The model under review builds one solid part; all positions refer to its coordinate system, in mm. A direction names the side the tool comes from. Coordinates: 2 decimals unless noted, no trailing zeros. Order: outer loops, then holes, each group sorted by start corner. A loop starts at its lowest first (then second) coordinate and runs counter-clockwise, first axis right, second up. Notation, with made-up numbers: (34.25, 35.25) - (88.25, 35.25) arc R16 cw to (88.25, 42.25) - close; hole circle Ø2 at (78.5, 9). An arc over 180 degrees is marked (long way). Answer in a Markdown table with one row per item.
```python
from build123d import *

# Parameters (mm, degrees)
F0_R     = 8.75
F0_R_2   = 4
F1_DEPTH = 21.3
F2_START = 3.8
F0_R_3   = 2.65
F2_DEPTH = 17.5
F4_DEPTH = 10


with BuildPart() as f1:
    # F0 (on Top) → F1 (new body)
    with BuildSketch(Plane.XY):
        Circle(F0_R)
        Circle(F0_R_2, mode=Mode.SUBTRACT)
    extrude(amount=F1_DEPTH)

    # F0 (on Top) → F2 (join)
    with BuildSketch(Plane.XY.offset(F2_START)):
        Circle(F0_R_2)
        Circle(F0_R_3, mode=Mode.SUBTRACT)
    extrude(amount=F2_DEPTH)

    # F3 (on face) → F4 (cut)
    with BuildSketch(Plane.XY.offset(21.3)):
        with BuildLine():
            ThreePointArc((-6.8053287944, -5.5), (0, -8.75), (6.8053287944, -5.5))
            Line((6.8053287944, -5.5), (-6.8053287944, -5.5))
        make_face()
        with BuildLine():
            Line((-6.8053287944, 5.5), (6.8053287944, 5.5))
            ThreePointArc((6.8053287944, 5.5), (0, 8.75), (-6.8053287944, 5.5))
        make_face()
    extrude(amount=-F4_DEPTH, mode=Mode.SUBTRACT)


solid = f1.part
```
Item 1: Mouldability with a two-part tool opening along Y and no side actions: class faces 4 (the face through (2.45, -1.01, 12.43)), 5 (the face through (4, -2, 0)), 6 (the face through (0, 5.5, 16)) as +Y half, -Y half, draft (parallel to the pull), parting line (faces both ways), or undercut.
Check values:
| item | result |
|---|---|
| face 4 | undercut |
| face 5 | draft |
| face 6 | +Y half |
Item 2: To check wall thickness, follow line 1 (Y direction, x = 0, z = 10.5); line 2 (Y direction, x = 0, z = 2.85); line 3 (X direction, y = 5.5, z = 7). State the ranges of each line that lie inside material, in increasing order. Write a range as from..to.
Check values:
| item | result |
|---|---|
| line 1 | -8.75..-2.65, 2.65..8.75 |
| line 2 | -8.75..-4, 4..8.75 |
| line 3 | -6.81..6.81 |
Item 3: Clearance check with flat-ended pins moving along their axes: pin 1 Ø1 at (x, z) = (2, 13.5) entering from -Y; pin 2 Ø4 at (x, y) = (1.5, 1) entering from -Z; pin 3 Ø1 at (x, z) = (1, 7) entering from -Y. State where each tip first meets the part, or that it passes through.
Check values:
| item | result |
|---|---|
| pin 1 | y = -5.5 |
| pin 2 | z = 3.8 |
| pin 3 | y = -8.74 |
Item 4: We need section C-C, the plane z = 13. Write out the cut boundary in (x, y), then the cut area to 3 significant figures.
Check values:
| item | result |
|---|---|
| outline | (-6.81, -5.5) - (6.81, -5.5) arc R8.75 ccw to (6.81, 5.5) - (-6.81, 5.5) arc R8.75 ccw to start; hole circle Ø5.3 at (0, 0) |
| area | 157 mm^2 |
Item 5: We need section B-B, the plane x = 0. Write out the cut boundary in (y, z).
Check values:
| item | result |
|---|---|
| outline | (-8.75, 0) - (-4, 0) - (-4, 3.8) - (-2.65, 3.8) - (-2.65, 21.3) - (-5.5, 21.3) - (-5.5, 11.3) - (-8.75, 11.3) - close; (2.65, 3.8) - (4, 3.8) - (4, 0) - (8.75, 0) - (8.75, 11.3) - (5.5, 11.3) - (5.5, 21.3) - (2.65, 21.3) - close |
Item 6: Tool access review of faces 1 (the face through (3, -1, 3.8)), 2 (the face through (0, -7, 11.3)), 3 (the face through (0, 7, 11.3)): name each direction out of +Z, -Z, +X, -X, +Y, -Y from which nothing blocks a thin tool from reaching the whole face with its end or side.
Check values:
| item | result |
|---|---|
| face 1 | -Z |
| face 2 | +Z, +X, -X, -Y |
| face 3 | +Z, +X, -X, +Y |
Item 7: We need section D-D, the plane x = 5.5. Write out the cut boundary in (y, z).
Check values:
| item | result |
|---|---|
| outline | (-6.81, 0) - (6.81, 0) - (6.81, 11.3) - (5.5, 11.3) - (5.5, 21.3) - (-5.5, 21.3) - (-5.5, 11.3) - (-6.81, 11.3) - close |
Item 8: We need section A-A, the plane y = 0. Write out the cut boundary in (x, z).
Check values:
| item | result |
|---|---|
| outline | (-8.75, 0) - (-4, 0) - (-4, 3.8) - (-2.65, 3.8) - (-2.65, 21.3) - (-8.75, 21.3) - close; (2.65, 3.8) - (4, 3.8) - (4, 0) - (8.75, 0) - (8.75, 21.3) - (2.65, 21.3) - close |
